Geometry check sheet. Reference: the model listing, model coordinates, mm. A direction names the side the tool comes from. Give positions to 0.01 mm unless a question says otherwise; leave off trailing zeros. Loops run counter-clockwise (first coordinate to the right, second up) from the corner with the lowest first, then second, coordinate; pieces in that order, holes last. Notation, with made-up numbers: (4, -38) -> (47, -38) arc R14 ccw to (47, -17) -> close; hole circle Ø3 at (9, -26). An arc over 180 degrees is marked (long way). Write each question's results on one line, items separated by ' | '. Start each with the question number.
1) Sectioned sample at C-C on z = 1.25. Record the cut outline in (x, y), then the cut area to 3 significant figures.
2) Sectioned sample at A-A on x = -1. Record the cut outline in (y, z).
3) Sectioned sample at B-B on y = 1. Record the cut outline in (x, z).
4) Set-up check for faces 4 (the face through (-1, 3, -0.597)), 5 (the face through (13.716, 5, 0)): record each of +Z, -Z, +X, -X, +Y, -Y from which the full face is reachable in a straight line by a thin tool's end or side.
5) Draft check along Z on faces 1 (the face through (0, 5, -9.004)), 2 (the face through (-0.597, 3, -1)), 3 (the face through (-13.716, 5, 0)). Enter one of: pulls with the +Z half, pulls with the -Z half, needs draft (parallel to the pull), parting line crosses it, or undercut.
6) Scan lines: line 1 (Z direction, x = -1, y = 1.5); line 2 (X direction, y = 0.5, z = 1.25); line 3 (X direction, y = 0.75, z = 0). Record each from-to range of solid material in increasing order. Write a range as from..to.
```python
from build123d import *

# Parameters (mm, degrees)
SKETCH1_W           = 27.432
SKETCH1_H           = 18.0086
BOSS_EXTRUDE1_DEPTH = 10.2616
CUT_EXTRUDE1_DEPTH  = 5.08


with BuildPart() as part:
    # Sketch1 → Boss-Extrude1 (new body)
    with BuildSketch(Plane(origin=(0, 0, 0), x_dir=(1, 0, 0), z_dir=(0, 1, 0))):
        Rectangle(SKETCH1_W, SKETCH1_H)
    extrude(amount=BOSS_EXTRUDE1_DEPTH)

    # Sketch2 → Cut-Extrude1 (cut)
    with BuildSketch(Plane.XZ):
        Polygon((-0.5969, 0.5969), (-0.5969, 1.9685), (0.5969, 1.9685), (0.5969, 0.5969), (1.9685, 0.5969), (1.9685, -0.5969), (0.5969, -0.5969), (0.5969, -1.9685), (-0.5969, -1.9685), (-0.5969, -0.5969), (-1.9685, -0.5969), (-1.9685, 0.5969), align=None)
    extrude(amount=-CUT_EXTRUDE1_DEPTH, mode=Mode.SUBTRACT)


solid = part.part
```
Result:
1) outline: (-13.72, 0) -> (-0.6, 0) -> (-0.6, 5.08) -> (0.6, 5.08) -> (0.6, 0) -> (13.72, 0) -> (13.72, 10.26) -> (-13.72, 10.26) -> close | area: 275 mm^2
2) outline: (0, -9) -> (10.26, -9) -> (10.26, 9) -> (0, 9) -> (0, 0.6) -> (5.08, 0.6) -> (5.08, -0.6) -> (0, -0.6) -> close
3) outline: (-13.72, -9) -> (13.72, -9) -> (13.72, 9) -> (-13.72, 9) -> close; hole (-1.97, -0.6) -> (-0.6, -0.6) -> (-0.6, -1.97) -> (0.6, -1.97) -> (0.6, -0.6) -> (1.97, -0.6) -> (1.97, 0.6) -> (0.6, 0.6) -> (0.6, 1.97) -> (-0.6, 1.97) -> (-0.6, 0.6) -> (-1.97, 0.6) -> close
4) face 4: -Y | face 5: +Z, -Z, +X, +Y, -Y
5) face 1: pulls with the -Z half | face 2: undercut | face 3: needs draft
6) line 1: -9..-0.6, 0.6..9 | line 2: -13.72..-0.6, 0.6..13.72 | line 3: -13.72..-1.97, 1.97..13.72
